Read the model definition and answer for the solid it produces. Units are mm, in the model's axes. A direction names the side the tool comes from. Give positions to 0.01 mm unless a question says otherwise; leave off trailing zeros. Order: outer loops, then holes, each group sorted by start corner. A loop starts at its lowest first (then second) coordinate and runs counter-clockwise, first axis right, second up. Notation, with made-up numbers: (63.5, 15) - (89.5, 15) arc R20 ccw to (89.5, 35) - close; hole circle Ø11 at (18, 66). An arc over 180 degrees is marked (long way). Answer as CSV lines item,"result". Start each with the question number.
Autodesk Inventor part; units mm, degrees
ref_plane "YZ Plane" through (0, 0, 0) normal (1, 0, 0) x (0, 1, 0)
ref_plane "XZ Plane" through (0, 0, 0) normal (0, 1, 0) x (-1, 0, 0)
ref_plane "XY Plane" through (0, 0, 0) normal (0, 0, 1) x (1, 0, 0)
sketch "Sketch1" plane through (0, 0, 0) normal (0, 1, 0) x (-1, 0, 0)
  line L0 (0, 0) -> (0, -22.8)
  line L1 (0, 0) -> (12.4, 0)
  line L2 (12.4, 0) -> (12.4, -22.8)
  line L3 (12.4, -22.8) -> (0, -22.8)
  line L4 (12.4, 0) -> (12.4, 1)
  line L5 (12.4, -22.8) -> (12.4, -23.8)
  line L6 (0, 0) -> (-1, 0)
  line L7 (12.4, 1) -> (-1, 1)
  line L8 (-1, 1) -> (-1, -23.8)
  line L9 (-1, -23.8) -> (12.4, -23.8)
  dimension "d0" = 22.8
  dimension "d1" = 12.4
  dimension "d2" = 1
  dimension "d3" = 1
extrude "Extrusion1" add sketch "Sketch1" along normal blind 21 contours L6 L8 L7 L4 L1 | L0 L3 L5 L9 L8 L6
sketch "Sketch2" plane through (-12.4, 0, -22.8) normal (0, 0, 1) x (1, 0, 0)
  line L0 (0, 0) -> (0, 21)
  line L1 (0, 0) -> (0, 1)
  line L2 (0, 1) -> (12.4, 1)
  line L3 (12.4, 0) -> (12.4, 21)
  line L4 (12.4, 0) -> (0, 0)
  dimension "d7" = 1
extrude "Extrusion2" add sketch "Sketch2" along normal blind 22.9
sketch "Sketch3" plane through (-12.4, 0, 1) normal (0, 0, 1) x (1, 0, 0)
  line L0 (12.4, 1) -> (0, 1)
  line L1 (0, 1) -> (0, 9)
  line L2 (0, 0) -> (0, 21)
  line L3 (0, 9) -> (13.4, 9)
  line L4 (13.4, 0) -> (13.4, 21)
  line L5 (13.4, 1) -> (13.4, 9)
  line L6 (13.4, 1) -> (0, 1)
  line L7 (0.5, 8.5) -> (0.5, 1.5)
  line L8 (0, 0) -> (13.4, 0)
  line L9 (0.5, 8.5) -> (12.9, 8.5)
  line L10 (12.4, 1) -> (12.4, 21)
  line L11 (12.9, 8.5) -> (12.9, 1.5)
  line L12 (12.9, 1.5) -> (0.5, 1.5)
  point P0 (12.4, 0)
  point P1 (12.4, 1.5)
  point P2 (12.4, 8.5)
  dimension "d10" = 8
extrude "Extrusion3" cut sketch "Sketch3" against normal blind 1 contours L12 L7 L9 L10
sketch "Sketch4" plane through (-12.4, 0, 1) normal (0, 0, 1) x (1, 0, 0)
  line L0 (12.4, 8.5) -> (0.5, 8.5)
  line L1 (2, 9.5) -> (2, 18.5)
  line L2 (2, 18.5) -> (0, 18.5)
  line L3 (0, 1) -> (0, 21)
  line L4 (2, 9.5) -> (0, 9.5)
  point P0 (12.4, 0)
  dimension "d20" = 9
extrude "Extrusion4" add sketch "Sketch4" along normal blind 7
sketch "Sketch5" plane through (1, 0, -23.8) normal (0, 0, -1) x (-1, 0, 0)
  line L0 (0, 0) -> (13.4, 0)
  line L1 (13.4, 0) -> (13.4, 9.398)
  line L2 (13.4, 0) -> (13.4, 21)
  line L3 (13.4, 9.398) -> (13.4, 18.3896)
  line L4 (13.4, 18.3896) -> (11.3934, 18.3896)
  line L5 (11.3934, 18.3896) -> (11.3934, 9.398)
  line L6 (11.3934, 9.398) -> (13.4, 9.398)
  point P0 (1, 0)
  dimension "d24" = 9.398
  dimension "d25" = 8.9916
  dimension "d26" = 2.0066
extrude "Extrusion5" add sketch "Sketch5" along normal blind 7
fillet "Fillet1" radius 3.175 4 edges at (-11.4, 18.5, 8) (-11.4, 9.5, 8) (-11.3967, 18.3896, -30.8) (-11.3967, 9.398, -30.8)
sketch "Sketch6" plane through (-10.4, 9.5, 1) normal (1, 0, 0) x (0, 0, -1)
  line L0 (0, 9) -> (-3.556, 9)
  line L1 (0, 9) -> (-3.825, 9)
  line L2 (-3.556, 9) -> (-3.556, 4.5042)
  line L3 (24.8, 8.8896) -> (28.625, 8.8896)
  circle A0 centre (-3.556, 4.5042) radius 2.413
  point P0 (1, -9.5)
  dimension "d33" = 3.556
  dimension "d34" = 4.4958
  dimension "d37" = 4.826
extrude "Extrusion6" cut sketch "Sketch6" against normal blind 7
thread "Thread1"
sketch "Sketch7" plane through (-10.3934, 9.398, -23.8) normal (1, 0, 0) x (0, 0, -1)
  line L0 (0, 8.9916) -> (3.556, 8.9916)
  line L1 (0, 8.9916) -> (3.825, 8.9916)
  line L2 (3.556, 8.9916) -> (3.556, 4.4958)
  circle A0 centre (3.556, 4.4958) radius 2.413
  point P0 (-23.8, -9.398)
  dimension "d42" = 3.556
  dimension "d43" = 4.4958
  dimension "d44" = 4.826
extrude "Extrusion7" cut sketch "Sketch7" against normal blind 7
thread "Thread2"
fillet "Fillet2" radius 1.524 4 edges at (-11.9, 8.5, 0.5) (0, 8.5, 0.5) (0, 1.5, 0.5) (-11.9, 1.5, 0.5)
properties part number "Servo Mount"
(1) Section D-D, the plane z = -17 is taken. Write down the section's boundary in (x, y), and give its area (3 significant figures).
(2) Flat-ended cylindrical pins translate along their axes: pin 1 Ø1 at (x, y) = (-11, 17) entering from +Z; pin 2 Ø0.6 at (x, z) = (-11, -25.5) entering from -Y; pin 3 Ø4 at (x, y) = (-6.5, 6) entering from -Z. Find the tip coordinate at first contact, or state that the pin passes through.
(3) Section A-A, the plane x = -3.5 is taken. Write down the section's boundary in (y, z).
(4) Section B-B, the plane z = -26 is taken. Write down the section's boundary in (x, y).
(5) Which of the six approach directions +Z, -Z, +X, -X, +Y, -Y give full straight-line access (tool end or side, diameter ignored) to faces 4 (the flat face through (-11, 9.5, 3)), 5 (the flat face through (-6, 11, -22.8)), 6 (the cylindrical face through (-11.442, 1.935, 0.493))?
(6) Determine the mould class of faces 1 (the cylindrical face through (-11.41, 10.35, -29.89)), 2 (the flat face through (-11, 14, 8)), 3 (the flat face through (-5.9, 1.5, 0.5)) for opening direction Y: released by +Y, released by -Y, zero draft, split by the parting line, or undercut.
(7) Section C-C, the plane y = 14.5 is taken. Write down the section's boundary in (x, z).
(8) Straight lines are drawn through the part: line 1 (Z direction, x = -5.5, y = 12); line 2 (X direction, y = 15.5, z = -18); line 3 (Z direction, x = -8.5, y = 7.25). For each, find the intervals that lie inside material, in ascending order. Write a range as [from, to].
Checks:
1,outline,"(-12.4, 0) - (1, 0) - (1, 21) - (0, 21) - (0, 1) - (-12.4, 1) - close"
1,area,"33.4 mm²"
2,pin 1,"stops at z = 7.77"
2,pin 2,"stops at y = 9.4"
2,pin 3,"stops at z = -23.8"
3,outline,"(0, -23.8) - (21, -23.8) - (21, -22.8) - (1, -22.8) - (1, 0) - (1.5, 0) - (1.5, 1) - (0, 1) - close; (8.5, 0) - (21, 0) - (21, 1) - (8.5, 1) - close"
4,outline,"(-12.4, 9.4) - (-10.39, 9.4) - (-10.39, 11.9) - (-12.4, 11.9) - close; (-12.4, 15.89) - (-10.39, 15.89) - (-10.39, 18.39) - (-12.4, 18.39) - close"
5,face 4,"+Z, +X, -X, -Y"
5,face 5,"-X, +Y"
5,face 6,"+Z"
6,face 1,"released by -Y"
6,face 2,"zero draft"
6,face 3,"undercut"
7,outline,"(-12.4, -30.8) - (-10.39, -30.8) - (-10.39, -29.69) - (-12.4, -29.69) - close; (-12.4, -25.02) - (-10.39, -25.02) - (-10.39, -23.8) - (1, -23.8) - (1, 1) - (-10.4, 1) - (-10.4, 2.19) - (-12.4, 2.19) - (-12.4, 0) - (0, 0) - (0, -22.8) - (-12.4, -22.8) - close; (-12.4, 6.92) - (-10.4, 6.92) - (-10.4, 8) - (-12.4, 8) - close"
8,line 1,"z = [-23.8, -22.8], [0, 1]"
8,line 2,"x = [0, 1]"
8,line 3,"z = [-23.8, -22.8]"
